```python
from build123d import *

# Parameters (mm, degrees)
SKETCH1_W           = 416
SKETCH1_H           = 166
BOSS_EXTRUDE1_DEPTH = 3
SKETCH2_W           = 30
SKETCH2_H           = 3.3
SKETCH2_W_2         = 3.5
SKETCH2_H_2         = 20
CUT_EXTRUDE1_DEPTH  = 3


with BuildPart() as part:
    # Sketch1 → Boss-Extrude1 (new body)
    with BuildSketch(Plane(origin=(0, 0, 0), x_dir=(1, 0, 0), z_dir=(0, 1, 0))):
        Rectangle(SKETCH1_W, SKETCH1_H)
    extrude(amount=BOSS_EXTRUDE1_DEPTH)

    # Sketch2 → Cut-Extrude1 (cut)
    with BuildSketch(Plane(origin=(0, 3, 0), x_dir=(1, 0, 0), z_dir=(0, 1, 0))):
        with Locations((-168, 81.35)):
            Rectangle(SKETCH2_W, SKETCH2_H)
        with Locations((-113, 81.35)):
            Rectangle(SKETCH2_W, SKETCH2_H)
        with Locations((-58, 81.35)):
            Rectangle(SKETCH2_W, SKETCH2_H)
        with Locations((-3, 81.35)):
            Rectangle(SKETCH2_W, SKETCH2_H)
        with Locations((52, 81.35)):
            Rectangle(SKETCH2_W, SKETCH2_H)
        with Locations((107, 81.35)):
            Rectangle(SKETCH2_W, SKETCH2_H)
        with Locations((162, 81.35)):
            Rectangle(SKETCH2_W, SKETCH2_H)
        with Locations((162, -81.35)):
            Rectangle(SKETCH2_W, SKETCH2_H)
        with Locations((107, -81.35)):
            Rectangle(SKETCH2_W, SKETCH2_H)
        with Locations((52, -81.35)):
            Rectangle(SKETCH2_W, SKETCH2_H)
        with Locations((-3, -81.35)):
            Rectangle(SKETCH2_W, SKETCH2_H)
        with Locations((-58, -81.35)):
            Rectangle(SKETCH2_W, SKETCH2_H)
        with Locations((-113, -81.35)):
            Rectangle(SKETCH2_W, SKETCH2_H)
        with Locations((-168, -81.35)):
            Rectangle(SKETCH2_W, SKETCH2_H)
        with Locations((-206.25, -34)):
            Rectangle(SKETCH2_W_2, SKETCH2_H_2)
        with Locations((-206.25, 0)):
            Rectangle(SKETCH2_W_2, SKETCH2_H_2)
        with Locations((-206.25, -68)):
            Rectangle(SKETCH2_W_2, SKETCH2_H_2)
        with Locations((-206.25, 34)):
            Rectangle(SKETCH2_W_2, SKETCH2_H_2)
        with Locations((-206.25, 68)):
            Rectangle(SKETCH2_W_2, SKETCH2_H_2)
        with Locations((206.25, -68)):
            Rectangle(SKETCH2_W_2, SKETCH2_H_2)
        with Locations((206.25, -34)):
            Rectangle(SKETCH2_W_2, SKETCH2_H_2)
        with Locations((206.25, 0)):
            Rectangle(SKETCH2_W_2, SKETCH2_H_2)
        with Locations((206.25, 34)):
            Rectangle(SKETCH2_W_2, SKETCH2_H_2)
        with Locations((206.25, 68)):
            Rectangle(SKETCH2_W_2, SKETCH2_H_2)
    extrude(amount=-CUT_EXTRUDE1_DEPTH, mode=Mode.SUBTRACT)


solid = part.part
```
CAD build for the part. Positions are in the model's coordinates, mm. Round coordinates to 2 decimals unless told otherwise and drop trailing zeros. Order: outer loops, then holes, each group sorted by start corner. A loop starts at its lowest first (then second) coordinate and runs counter-clockwise, first axis right, second up.
Item 1: Saw through at B-B on x = -102. Write the cut outline in (y, z), then the cut area to 3 significant figures.
Item 2: Saw through at A-A on z = -40. Write the cut outline in (x, y).
Item 3: Probe line 1 along X through (y, z) = (1.8, 65.5); line 2 along Z through (x, y) = (-46, 1.45). List the from-to ranges inside material, lowest first.
Item 4: Pin check, flat tips, straight feed: pin 1 (1.5 mm diameter, centred on x = 159.5, y = 2, fed in from -Z); pin 2 (1.5 mm diameter, centred on y = 1, z = -65, fed in from +X); pin 3 (1 mm diameter, centred on x = -52, y = 2, fed in from +Z). Stop position of each tip, or through.
Reported:
1. outline: (0, -79.7) - (3, -79.7) - (3, 79.7) - (0, 79.7) - close
1. area: 478 mm2
2. outline: (-204.5, 0) - (204.5, 0) - (204.5, 3) - (-204.5, 3) - close
3. line 1: x = -204.5 to 204.5
3. line 2: z = -79.7 to 79.7
4. pin 1: stops at z = -79.7
4. pin 2: stops at x = 204.5
4. pin 3: stops at z = 79.7
